The listing builds one solid part. Answer for the finished solid, in the listing's coordinates (mm). Round coordinates to 2 decimals unless told otherwise and drop trailing zeros. Write each loop counter-clockwise with the first axis right and the second up, starting at its lowest first coordinate (ties: lowest second). Pieces come first, ordered by that corner, then holes. Notation, with made-up numbers: (28, -29) - (37, -29) arc R6 cw to (37, -23) - close; hole circle Ø8 at (1.5, 58.5). An arc over 180 degrees is marked (long way). Answer in a Markdown table with one row per item.
from build123d import *

# Parameters (mm, degrees)
SKETCH_1_R           = 175
EXTRUDE_1_DEPTH      = 3
CUT_EXTRUDE_1_DEPTH  = 3
FILLET_1_R           = 5
FILLET_2_R           = 5
FILLET_3_R           = 5
SKETCH_5_R           = 1.5
CUT_EXTRUDE_4_DEPTH  = 3
SKETCH_6_R           = 1.5
CUT_EXTRUDE_5_DEPTH  = 3
SKETCH_7_W           = 30
SKETCH_7_H           = 108
CUT_EXTRUDE_6_DEPTH  = 3
SKETCH_8_R           = 1.5
CUT_EXTRUDE_7_DEPTH  = 3
SKETCH_9_R           = 1.5
CUT_EXTRUDE_8_DEPTH  = 10
SKETCH_10_R          = 1.6
CUT_EXTRUDE_9_DEPTH  = 10
SKETCH_11_W          = 15
SKETCH_11_H          = 30
CUT_EXTRUDE_10_DEPTH = 10
SKETCH_22_R          = 1.5
CUT_EXTRUDE_11_DEPTH = 10
SKETCH_23_R          = 1.5
CUT_EXTRUDE_12_DEPTH = 10


with BuildPart() as part:
    # ｽｹｯﾁ1 → ﾎﾞｽ - 押し出し1 (new body)
    with BuildSketch(Plane.XY):
        Circle(SKETCH_1_R)
    extrude(amount=EXTRUDE_1_DEPTH)

    # ｽｹｯﾁ2 → ｶｯﾄ - 押し出し1 (cut)
    with BuildSketch(Plane.XY.offset(3)):
        with BuildLine():
            Line((-60, 115), (0, 115))
            Line((0, 115), (0, 175))
            ThreePointArc((0, 175), (-30.465194158, 172.327803749), (-60, 164.392822228))
            Line((-60, 164.392822228), (-60, 115))
        make_face()
        with BuildLine():
            Line((0, 175), (0, 115))
            Line((0, 115), (60, 115))
            Line((60, 115), (60, 164.392822228))
            ThreePointArc((60, 164.392822228), (30.465194158, 172.327803749), (0, 175))
        make_face()
        with BuildLine():
            Line((0, -175), (0, -115))
            Line((0, -115), (-60, -115))
            Line((-60, -115), (-60, -164.392822228))
            ThreePointArc((-60, -164.392822228), (-30.465194158, -172.327803749), (0, -175))
        make_face()
        with BuildLine():
            Line((60, -115), (0, -115))
            Line((0, -115), (0, -175))
            ThreePointArc((0, -175), (30.465194158, -172.327803749), (60, -164.392822228))
            Line((60, -164.392822228), (60, -115))
        make_face()
    extrude(amount=-CUT_EXTRUDE_1_DEPTH, mode=Mode.SUBTRACT)

    # ﾌｨﾚｯﾄ1
    fillet_1_edges = [part.edges().sort_by_distance(p)[0] for p in [
        (-60, 164.392822228, 1.5),
    ]]
    fillet(fillet_1_edges, radius=FILLET_1_R)

    # ﾌｨﾚｯﾄ2
    fillet_2_edges = [part.edges().sort_by_distance(p)[0] for p in [
        (-60, 115, 1.5),
        (60, 164.392822228, 1.5),
        (60, 115, 1.5),
    ]]
    fillet(fillet_2_edges, radius=FILLET_2_R)

    # ﾌｨﾚｯﾄ3
    fillet_3_edges = [part.edges().sort_by_distance(p)[0] for p in [
        (-60, -115, 1.5),
        (60, -115, 1.5),
        (60, -164.392822228, 1.5),
        (-60, -164.392822228, 1.5),
    ]]
    fillet(fillet_3_edges, radius=FILLET_3_R)

    # ｽｹｯﾁ5 → ｶｯﾄ - 押し出し4 (cut)
    with BuildSketch(Plane.XY.offset(3)):
        with Locations((-100, -115)):
            Circle(SKETCH_5_R)
        with Locations((100, -115)):
            Circle(SKETCH_5_R)
        with Locations((100, 115)):
            Circle(SKETCH_5_R)
        with Locations((-100, 115)):
            Circle(SKETCH_5_R)
    extrude(amount=-CUT_EXTRUDE_4_DEPTH, mode=Mode.SUBTRACT)

    # ｽｹｯﾁ6 → ｶｯﾄ - 押し出し5 (cut)
    with BuildSketch(Plane.XY.offset(3)):
        with Locations((-60, 54)):
            Circle(SKETCH_6_R)
        with Locations((60, 54)):
            Circle(SKETCH_6_R)
        with Locations((-60, -54)):
            Circle(SKETCH_6_R)
        with Locations((60, -54)):
            Circle(SKETCH_6_R)
    extrude(amount=-CUT_EXTRUDE_5_DEPTH, mode=Mode.SUBTRACT)

    # ｽｹｯﾁ7 → ｶｯﾄ - 押し出し6 (cut)
    with BuildSketch(Plane.XY.offset(3)):
        with Locations((-85, 0)):
            Rectangle(SKETCH_7_W, SKETCH_7_H)
    extrude(amount=-CUT_EXTRUDE_6_DEPTH, mode=Mode.SUBTRACT)

    # ｽｹｯﾁ8 → ｶｯﾄ - 押し出し7 (cut)
    with BuildSketch(Plane.XY.offset(3)):
        with Locations((-115, -67)):
            Circle(SKETCH_8_R)
        with Locations((-116.822468618, 0)):
            Circle(SKETCH_8_R)
        with Locations((-115, 67)):
            Circle(SKETCH_8_R)
    extrude(amount=-CUT_EXTRUDE_7_DEPTH, mode=Mode.SUBTRACT)

    # ｽｹｯﾁ9 → ｶｯﾄ - 押し出し8 (cut)
    with BuildSketch(Plane.XY.offset(3)):
        with Locations((-65, 37)):
            Circle(SKETCH_9_R)
        with Locations((20, 41)):
            Circle(SKETCH_9_R)
        with Locations((-65, -38)):
            Circle(SKETCH_9_R)
        with Locations((20, -40)):
            Circle(SKETCH_9_R)
    extrude(amount=-CUT_EXTRUDE_8_DEPTH, mode=Mode.SUBTRACT)

    # ｽｹｯﾁ10 → ｶｯﾄ - 押し出し9 (cut)
    with BuildSketch(Plane.XY.offset(3)):
        with Locations((111.643659725, -125.921059639)):
            Circle(SKETCH_10_R)
        with Locations((122.679794489, -115.037952538)):
            Circle(SKETCH_10_R)
        with Locations((168, 7.75)):
            Circle(SKETCH_10_R)
        with Locations((168, -7.75)):
            Circle(SKETCH_10_R)
        with Locations((111.56768007, 125.844011632)):
            Circle(SKETCH_10_R)
        with Locations((122.679794489, 115.037952538)):
            Circle(SKETCH_10_R)
    extrude(amount=-CUT_EXTRUDE_9_DEPTH, mode=Mode.SUBTRACT)

    # ｽｹｯﾁ11 → ｶｯﾄ - 押し出し10 (cut)
    with BuildSketch(Plane.XY.offset(3)):
        with Locations((81.317279836, 81.317279836)):
            Rectangle(SKETCH_11_W, SKETCH_11_H)
        with Locations((81.317279836, -81.317279836)):
            Rectangle(SKETCH_11_W, SKETCH_11_H)
    extrude(amount=-CUT_EXTRUDE_10_DEPTH, mode=Mode.SUBTRACT)

    # ｽｹｯﾁ22 → ｶｯﾄ - 押し出し11 (cut)
    with BuildSketch(Plane.XY.offset(10)):
        with Locations((150, -10)):
            Circle(SKETCH_22_R)
        with Locations((150, 10)):
            Circle(SKETCH_22_R)
    extrude(amount=-CUT_EXTRUDE_11_DEPTH, mode=Mode.SUBTRACT)

    # ｽｹｯﾁ23 → ｶｯﾄ - 押し出し12 (cut)
    with BuildSketch(Plane.XY.offset(3)):
        with Locations((80, 145)):
            Circle(SKETCH_23_R)
        with Locations((80, 129.5)):
            Circle(SKETCH_23_R)
        with Locations((80, -129.5)):
            Circle(SKETCH_23_R)
        with Locations((80, -145)):
            Circle(SKETCH_23_R)
        with Locations((-140, 37.5)):
            Circle(SKETCH_23_R)
        with Locations((-140, -37.5)):
            Circle(SKETCH_23_R)
    extrude(amount=-CUT_EXTRUDE_12_DEPTH, mode=Mode.SUBTRACT)


solid = part.part
(1) Flat-ended cylindrical pins translate along their axes: pin 1 (0.9 mm diameter, centred on y = 11.5, z = 1.5, fed in from -X); pin 2 (2 mm diameter, centred on x = 36, y = 67, fed in from -Z); pin 3 (0.9 mm diameter, centred on x = -16.5, z = 1, fed in from +Y); pin 4 (1 mm diameter, centred on x = -70.5, z = 1, fed in from -Y). Find the tip coordinate at first contact, or state that the pin passes through.
Checked values:
| item | result |
|---|---|
| pin 1 | stops at x = -174.65 |
| pin 2 | stops at z = 0 |
| pin 3 | stops at y = 115 |
| pin 4 | stops at y = -160.39 |
(2) Section B-B (z = 2.5) is taken. State how many separate pieces and enclosed holes the cut face has, and give its area (3 significant figures).
Checked values:
| item | result |
|---|---|
| separate pieces | 1 |
| enclosed holes | 32 |
| area | 78,300 mm2 |
(3) Find the intervals of material crossed by line 1 (Y direction, x = -65, z = 0.75); line 2 (X direction, y = -67, z = 1); line 3 (Y direction, x = -139, z = 1.25), in increasing order.
Checked values:
| item | result |
|---|---|
| line 1 | y = -162.08 to -39.5, -36.5 to 35.5, 38.5 to 162.08 |
| line 2 | x = -161.67 to -116.5, -113.5 to 73.82, 88.82 to 161.67 |
| line 3 | y = -106.32 to -38.62, -36.38 to 36.38, 38.62 to 106.32 |
(4) Section A-A (x = -76.5) is taken. Give the vertices of the cut face in (y, z), and give its area (3 significant figures).
Checked values:
| item | result |
|---|---|
| outline | (-157.39, 0) - (-54, 0) - (-54, 3) - (-157.39, 3) - close; (54, 0) - (157.39, 0) - (157.39, 3) - (54, 3) - close |
| area | 620 mm2 |
(5) Section C-C (y = 104) is taken. Give the vertices of the cut face in (x, z).
Checked values:
| item | result |
|---|---|
| outline | (-140.74, 0) - (140.74, 0) - (140.74, 3) - (-140.74, 3) - close |
